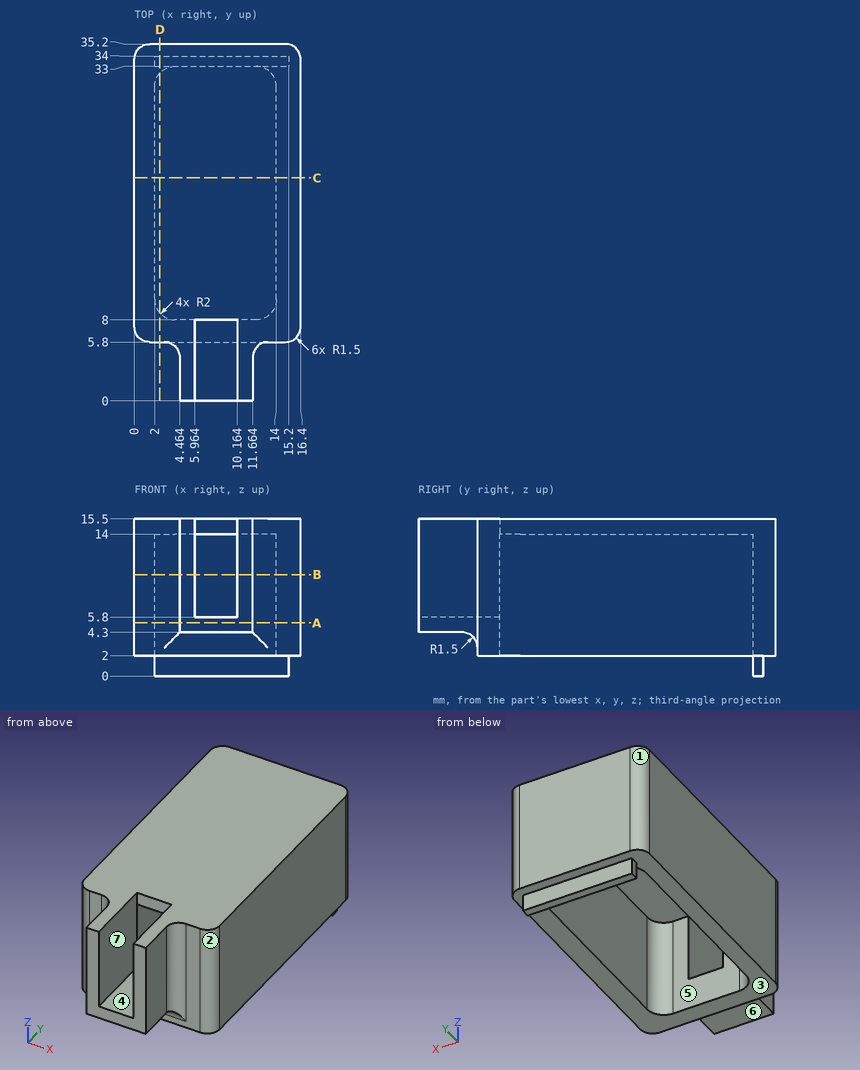
Design review of the part shown in the three views and the two pictorial views. Dimensions are in mm from the part's minimum x, y and z. A direction names the side the tool comes from. Coordinates: 2 decimals unless noted, no trailing zeros. Write each loop counter-clockwise with the first axis right and the second up, starting at its lowest first coordinate (ties: lowest second). Pieces come first, ordered by that corner, then holes.
1) Clearance check with flat-ended pins moving along their axes: pin 1 Ø1.3 at (x, y) = (8, 2) entering from +Z; pin 2 Ø0.8 at (y, z) = (33.5, 0.5) entering from +X; pin 3 Ø4.5 at (y, z) = (3, 11) entering from -X (1 decimal). State where each tip first meets the part, or that it passes through.
2) We need section B-B on z = 10. State the section outline as (x, y) points, then the cut area to 3 significant figures.
3) Machinability: for the marked faces 5, 6 and 7, which of the approach directions +Z, -Z, +X, -X, +Y, -Y give a long, thin tool a straight path to every point of the face, cutting with its end or side? Answer none if there is none.
4) We need section D-D on x = 2.5. State the section outline as (y, z) points.
5) The part is to be moulded in two halves that separate along X. For the marked faces 1, 2, 3 and 4, say which applies: pulls with the +X half, pulls with the -X half, needs draft (parallel to the pull), parting line crosses it, or undercut.
6) We need section A-A on z = 5.25. State the section outline as (x, y) points, then the cut area to 3 significant figures.
7) We need section C-C on y = 22. State the section outline as (x, z) points, then the cut area to 3 significant figures.
8) To check wall thickness, follow probe 1 along X at (y, z) = (17.5, 2.75); probe 2 along Y at (x, z) = (5, 12); probe 3 along Y at (x, z) = (11.5, 2.25). State the ranges of each line that lie inside material, in increasing order.
Answer list:
1. pin 1: stops at z = 5.8
1. pin 2: stops at x = 15.2
1. pin 3: stops at x = 4.1
2. outline: (0, 7.3) arc R1.5 ccw to (1.5, 5.8) - (2.96, 5.8) arc R1.5 cw to (4.46, 4.3) - (4.46, 0) - (5.96, 0) - (5.96, 8) - (4, 8) arc R2 cw to (2, 10) - (2, 31) arc R2 cw to (4, 33) - (12, 33) arc R2 cw to (14, 31) - (14, 10) arc R2 cw to (12, 8) - (10.16, 8) - (10.16, 0) - (11.66, 0) - (11.66, 4.3) arc R1.5 cw to (13.16, 5.8) - (14.9, 5.8) arc R1.5 ccw to (16.4, 7.3) - (16.4, 33.7) arc R1.5 ccw to (14.9, 35.2) - (1.5, 35.2) arc R1.5 ccw to (0, 33.7) - close
2. area: 193 mm2
3. face 5: -Z
3. face 6: -Z, +X, -X, -Y
3. face 7: +Z, -Y
4. outline: (5.8, 2) - (8.68, 2) - (8.68, 14) - (32.32, 14) - (32.32, 2) - (33, 2) - (33, 0) - (34, 0) - (34, 2) - (35.2, 2) - (35.2, 15.5) - (5.8, 15.5) - close
5. face 1: pulls with the -X half
5. face 2: pulls with the +X half
5. face 3: needs draft
5. face 4: undercut
6. outline: (0, 7.3) arc R1.5 ccw to (1.5, 5.8) - (2.96, 5.8) arc R1.5 cw to (4.46, 4.3) - (4.46, 0) - (11.66, 0) - (11.66, 4.3) arc R1.5 cw to (13.16, 5.8) - (14.9, 5.8) arc R1.5 ccw to (16.4, 7.3) - (16.4, 33.7) arc R1.5 ccw to (14.9, 35.2) - (1.5, 35.2) arc R1.5 ccw to (0, 33.7) - close; hole (2, 10) arc R2 ccw to (4, 8) - (12, 8) arc R2 ccw to (14, 10) - (14, 31) arc R2 ccw to (12, 33) - (4, 33) arc R2 ccw to (2, 31) - close
6. area: 226 mm2
7. outline: (0, 2) - (2, 2) - (2, 14) - (14, 14) - (14, 2) - (16.4, 2) - (16.4, 15.5) - (0, 15.5) - close
7. area: 77.4 mm2
8. probe 1: x = 0 to 2, 14 to 16.4
8. probe 2: y = 0 to 8, 33 to 35.2
8. probe 3: y = 5.8 to 8, 33 to 35.2
